Geometry check sheet. Reference: the model listing, model coordinates, mm. A direction names the side the tool comes from. Coordinates: 2 decimals unless noted, no trailing zeros. Write each loop counter-clockwise with the first axis right and the second up, starting at its lowest first coordinate (ties: lowest second). Pieces come first, ordered by that corner, then holes. Notation, with made-up numbers: M 18.5,-9.75 L 67.5,-9.75 A26 cw 67.5,5.25 Z; hole C 19.25,-3 d8. An arc over 180 degrees is marked long. Write item = value, one per line. Start each with the question number.
```python
from build123d import *

# Parameters (mm, degrees)
SALIENTE_EXTRUIR1_DEPTH = 12
SALIENTE_EXTRUIR2_DEPTH = 2.5
REDONDEO2_R             = 0.5
SALIENTE_EXTRUIR4_DEPTH = 14.5
REDONDEO5_R             = 1


with BuildPart() as part:
    # Croquis1 → Saliente-Extruir1 (new body)
    with BuildSketch(Plane(origin=(0, 0, 0), x_dir=(1, 0, 0), z_dir=(0, 1, 0))):
        Polygon((8.602519010925427, 1.1e-16), (4.301259505462714, 7.45), (-4.30125950546271, 7.450000000000001), (-8.602519010925425, 1.1e-16), (-4.301259505462709, -7.450000000000002), (4.301259505462713, -7.450000000000001), align=None)
        Polygon((-3.723909236273085, 6.45), (-7.447818472546173, 8.7e-16), (-3.723909236273083, -6.450000000000002), (3.723909236273086, -6.450000000000001), (7.4478184725461745, 0), (3.7239092362730872, 6.45), align=None, mode=Mode.SUBTRACT)
    extrude(amount=SALIENTE_EXTRUIR1_DEPTH)

    # Croquis2 → Saliente-Extruir2 (add)
    with BuildSketch(Plane.XZ):
        Polygon((8.602519010925427, -1.1e-16), (4.301259505462713, 7.450000000000001), (-4.301259505462709, 7.450000000000002), (-8.602519010925425, -1.1e-16), (-4.30125950546271, -7.450000000000001), (4.301259505462714, -7.45), align=None)
    extrude(amount=SALIENTE_EXTRUIR2_DEPTH)

    # Redondeo2
    redondeo2_edges = [part.edges().sort_by_distance(p)[0] for p in [
        (8.9e-16, 12, -6.45),
        (-5.585863854409629, 12, -3.2250000000000005),
        (-5.585863854409627, 12, 3.2250000000000005),
        (1.78e-15, 12, 6.450000000000001),
        (5.585863854409631, 12, 3.2250000000000005),
        (5.585863854409631, 12, -3.225),
    ]]
    fillet(redondeo2_edges, radius=REDONDEO2_R)

    # Croquis3 → Saliente-Extruir4 (add)
    with BuildSketch(Plane.XZ.offset(2.5)):
        with BuildLine():
            Line((4.301259505462713, 7.450000000000002), (8.602519010925427, -1.1e-16))
            ThreePointArc((8.602519010925423, 0), (7.45, 4.301259505462711), (4.3012595054627125, 7.449999999999999))
        make_face()
        with BuildLine():
            ThreePointArc((4.3012595054627125, 7.449999999999999), (5.3e-16, 8.602519010925423), (-4.30125950546271, 7.45))
            Line((-4.30125950546271, 7.450000000000002), (4.301259505462713, 7.450000000000001))
        make_face()
        with BuildLine():
            ThreePointArc((-4.30125950546271, 7.45), (-7.449999999999998, 4.301259505462714), (-8.602519010925423, 1.05e-15))
            Line((-8.602519010925425, 0), (-4.301259505462709, 7.450000000000002))
        make_face()
        with BuildLine():
            ThreePointArc((-8.602519010925423, 1.05e-15), (-7.449999999999999, -4.3012595054627125), (-4.301259505462708, -7.450000000000001))
            Line((-4.30125950546271, -7.450000000000001), (-8.602519010925425, -1.1e-16))
        make_face()
        with BuildLine():
            Line((4.301259505462713, -7.45), (-4.30125950546271, -7.450000000000001))
            ThreePointArc((-4.301259505462708, -7.450000000000001), (-1.58e-15, -8.602519010925423), (4.3012595054627125, -7.449999999999999))
        make_face()
        with BuildLine():
            Line((8.602519010925427, 0), (4.301259505462714, -7.45))
            ThreePointArc((4.3012595054627125, -7.449999999999999), (7.450000000000001, -4.301259505462709), (8.602519010925423, -2.11e-15))
        make_face()
    extrude(amount=-SALIENTE_EXTRUIR4_DEPTH)

    # Redondeo5
    redondeo5_edges = [part.edges().sort_by_distance(p)[0] for p in [
        (8.602519010925413, -2.5, 5.94e-15),
    ]]
    fillet(redondeo5_edges, radius=REDONDEO5_R)


solid = part.part
```
Q1. Draft check along X on faces 1 (the face through (0, -2.5, 0)), 2 (the face through (0, 6, -6.45)), 3 (the face through (1.86, 5.16, 8.4)). Enter one of: pulls with the +X half, pulls with the -X half, needs draft (parallel to the pull), parting line crosses it, or undercut.
Q2. Scan lines: L1, parallel to Y at x = -1, z = 2; L2, parallel to Z at x = -0.5, y = 2; L3, parallel to X at y = 5.25, z = -3.5. Record each from-to range of solid material in increasing order.
Q3. Cross-section at B-B on x = 0. Enter the section's corners in (y, z), and give its area (3 significant figures).
Q4. Cross-section at C-C on y = -1. Enter the section's corners in (x, z), and give its area (3 significant figures).
Q5. Cross-section at A-A on y = 0.5. Enter the section's corners in (x, z), and give its area (3 significant figures).
Q6. Gauge pin test, flat ends, axial feed: pin 1 (6.5 mm diameter, centred on x = 3.5, z = 1, fed in from +Y); pin 2 (2 mm diameter, centred on x = -2.5, y = 4, fed in from +Z); pin 3 (2 mm diameter, centred on x = -1.5, y = 6.5, fed in from +Z). Record the tip position at first contact, or that the pin passes through.
Q7. Set-up check for faces 4 (the face through (5.69, 11.86, -3.35)), 5 (the face through (-6.41, 12, -3.15)): record each of +Z, -Z, +X, -X, +Y, -Y from which the full face is reachable in a straight line by a thin tool's end or side.
Values found:
q1.face_1 = needs draft
q1.face_2 = undercut
q1.face_3 = parting line crosses it
q2.L1 = -2.5 to 0
q2.L2 = -8.59 to -6.45, 6.45 to 8.59
q2.L3 = -7.86 to -5.43, 5.43 to 7.86
q3.outline = M -2.5,-7.6 A1 ccw -1.5,-8.6 L 12,-8.6 L 12,-6.95 A0.5 ccw 11.5,-6.45 L 0,-6.45 L 0,6.45 L 11.5,6.45 A0.5 ccw 12,6.95 L 12,8.6 L -1.5,8.6 A1 ccw -2.5,7.6 Z
q3.area = 94.1 mm²
q4.outline = C 0,0 d17.21
q4.area = 232 mm²
q5.outline = C 0,0 d17.21; hole M -7.45,0 L -3.72,-6.45 L 3.72,-6.45 L 7.45,0 L 3.72,6.45 L -3.72,6.45 Z
q5.area = 88.4 mm²
q6.pin_1 = 11.97
q6.pin_2 = 8.47
q6.pin_3 = 8.59
q7.face_4 = +Y
q7.face_5 = +Z, -Z, +X, -X, +Y
